Can you work these out from the model? Positions are in its coordinate system, mm. Face numbers are marked on the shaded views. A direction names the side the tool comes from. Give positions to 0.01 mm unless a question says otherwise; leave off trailing zeros. Order: outer loops, then holes, each group sorted by start corner. A loop starts at its lowest first (then second) coordinate and runs counter-clockwise, first axis right, second up. Notation, with made-up numbers: M 48,43 L 61,43 A29 ccw 61,72 Z; hole C 22,-34 d4. An arc over 180 degrees is marked long. Write each question's results on one line, items separated by ' | '.
from build123d import *

# Parameters (mm, degrees)
AUFSATZ_LINEAR_AUSTRAGEN1_DEPTH                      = 6
FORMSENKUNG_F_R_M4_SENKSCHRAUBE_MIT_INNE_D           = 4.8
FORMSENKUNG_F_R_M4_SENKSCHRAUBE_MIT_INNE_CSINK_D     = 11.18
FORMSENKUNG_F_R_M4_SENKSCHRAUBE_MIT_INNE_CSINK_ANGLE = 90
AUFSATZ_LINEAR_AUSTRAGEN2_DEPTH                      = 60
AUFSATZ_LINEAR_AUSTRAGEN2_DEPTH_BACK                 = 6
STIRNSENKUNG_F_R_1_4_FLACHKOPFSCHRAUBE_D             = 7.14248
STIRNSENKUNG_F_R_1_4_FLACHKOPFSCHRAUBE_CBORE_D       = 11.90752
STIRNSENKUNG_F_R_1_4_FLACHKOPFSCHRAUBE_CBORE_DEPTH   = 0.500000016


with BuildPart() as part:
    # Skizze1 → Aufsatz-Linear austragen1 (new body)
    with BuildSketch(Plane.XY):
        with BuildLine():
            Line((-15, 12), (-15, 3))
            ThreePointArc((-15, 3), (-14.121320344, 0.878679656), (-12, 0))
            Line((-12, 0), (12, 0))
            ThreePointArc((12, 0), (14.121320344, 0.878679656), (15, 3))
            Line((15, 3), (15, 12))
            ThreePointArc((15, 12), (0, 13.905249807), (-15, 12))
        make_face()
    extrude(amount=AUFSATZ_LINEAR_AUSTRAGEN1_DEPTH)

    # Formsenkung für M4 Senkschraube mit Innensechskant1 (through all)
    with Locations(Plane.XY.offset(6)):
        with Locations((-8, 6.4), (8, 6.4)):
            CounterSinkHole(FORMSENKUNG_F_R_M4_SENKSCHRAUBE_MIT_INNE_D / 2, FORMSENKUNG_F_R_M4_SENKSCHRAUBE_MIT_INNE_CSINK_D / 2, counter_sink_angle=FORMSENKUNG_F_R_M4_SENKSCHRAUBE_MIT_INNE_CSINK_ANGLE)

    # Skizze4 → Aufsatz-Linear austragen2 (add, two sides)
    with BuildSketch(Plane.XY.offset(6)) as aufsatz_linear_austragen2_sk:
        with BuildLine():
            Line((-15, 12), (-15, 23))
            Line((-15, 23), (15, 23))
            Line((15, 23), (15, 12))
            ThreePointArc((15, 12), (0, 13.905249807), (-15, 12))
        make_face()
    extrude(amount=AUFSATZ_LINEAR_AUSTRAGEN2_DEPTH)
    extrude(aufsatz_linear_austragen2_sk.sketch, amount=-AUFSATZ_LINEAR_AUSTRAGEN2_DEPTH_BACK)

    # Stirnsenkung für 1/4 Flachkopfschraube (Kopf Button)1 (through all)
    with Locations(Plane(origin=(0.121475485, 13.905126838, 38.119269102), x_dir=(-0.999997951, 0.002024591, 0), z_dir=(-0.002024591, -0.999997951, 0))):
        with Locations((0, 0)):
            CounterBoreHole(STIRNSENKUNG_F_R_1_4_FLACHKOPFSCHRAUBE_D / 2, STIRNSENKUNG_F_R_1_4_FLACHKOPFSCHRAUBE_CBORE_D / 2, STIRNSENKUNG_F_R_1_4_FLACHKOPFSCHRAUBE_CBORE_DEPTH)


solid = part.part
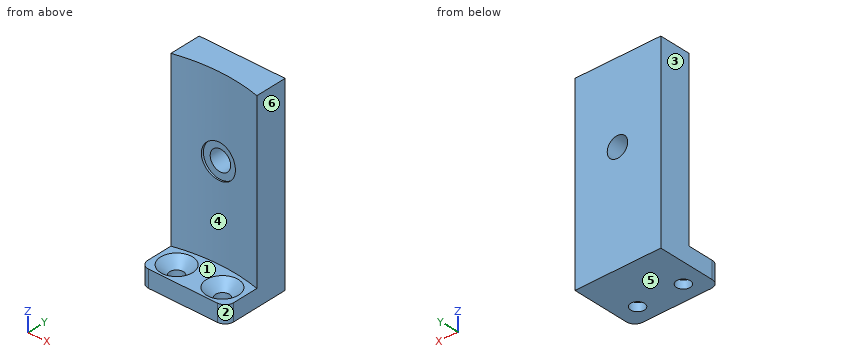
(1) Imagine slicing it at C-C, the plane z = 52.5. Write out the boundary of the cut face in (x, y), plus the area to 3 significant figures.
Data:
outline: M -15,12 A60 cw 15,12 L 15,23 L -15,23 Z | area: 292 mm2
(2) I need wall thicknesses on L1, parallel to X at y = 6.4, z = 1.25; L2, parallel to Y at x = -8, z = 1.05; L3, parallel to Z at x = 3, y = 10. Which ranges of each line are inside material? Lowest first, please. Write a range as from..to.
Data:
L1: x = -15..-10.4, -5.6..5.6, 10.4..15 | L2: y = 0..4, 8.8..23 | L3: z = 0..6
(3) Imagine slicing it at B-B, the plane x = 8. Write out the boundary of the cut face in (y, z).
Data:
outline: M 0,0 L 4,0 L 4,2.81 L 0.81,6 L 0,6 Z; M 8.8,0 L 23,0 L 23,66 L 13.37,66 L 13.37,6 L 11.99,6 L 8.8,2.81 Z
(4) We'd pull the mould along X, two halves only. Please class the marked faces 3, 4, 5 and 6: +X half, -X half, draft (parallel to the pull), parting line (faces both ways), or undercut.
Data:
face 3: -X half | face 4: undercut | face 5: draft | face 6: +X half
(5) Imagine slicing it at A-A, the plane y = 6.4. Write out the boundary of the cut face in (x, z).
Data:
outline: M -15,0 L -10.4,0 L -10.4,2.81 L -13.59,6 L -15,6 Z; M -5.6,0 L 5.6,0 L 5.6,2.81 L 2.41,6 L -2.41,6 L -5.6,2.81 Z; M 10.4,0 L 15,0 L 15,6 L 13.59,6 L 10.4,2.81 Z
(6) For the marked faces 1 and 2, which set-ups out of +Z, -Z, +X, -X, +Y, -Y let a thin tool reach every point of the face, with its end or its side?
Data:
face 1: +Z, -Y | face 2: +Z, -Z, +X, -Y
(7) Will these pins go through, and if not, where does the flat tip stop? P1, Ø4, axis at x = 0.5, y = 10, coming from the +Z side; P2, Ø1.5, axis at x = 7.5, y = 4, coming from the -Z side.
Data:
P1: stops at z = 6 | P2: stops at z = 0
